Can you work these out from the drawing? Everything is in mm from the part's minimum corner. Give positions to 0.01 mm unless a question says otherwise; leave off trailing zeros. Write each loop counter-clockwise with the first axis right and the second up, starting at its lowest first coordinate (ties: lowest second). Pieces come first, ordered by that corner, then holes. Notation, with made-up numbers: (-3, 71) -> (27, 71) arc R21 ccw to (27, 92) -> close; hole circle Ø11 at (18.5, 59). An arc over 180 degrees is marked (long way). Use one line per item in the form item = value.
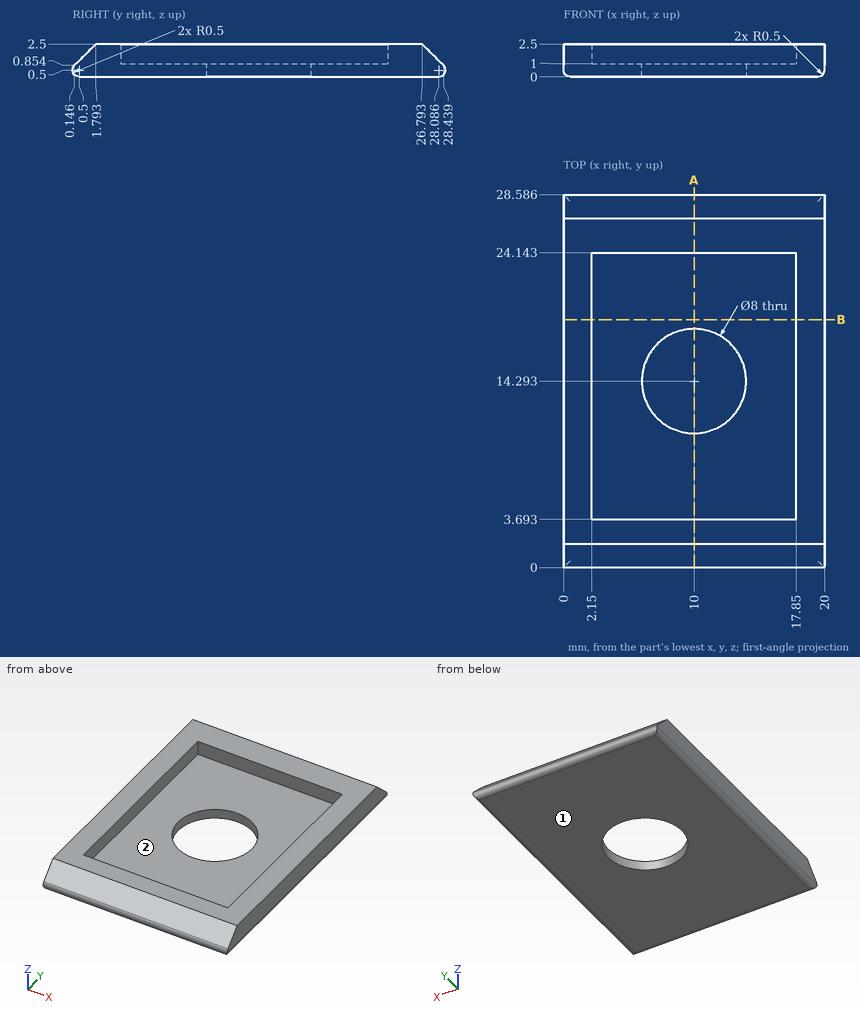
Q1. If we mould it in two halves opening along X, with no side actions, what happens to the marked faces 1 and 2? For each: +X half, -X half, draft (parallel to the pull), parting line (faces both ways), or undercut.
Result set:
face_1 = draft
face_2 = undercut
Q2. If I drill on line 1 along X through (y, z) = (7.75, 1.4); line 2 along Y through (x, z) = (10, 0.45); line 3 along Y through (x, z) = (10, 0.85) (1 decimal), over which ranges is the centre line in solid material (lowest first)? Write a range as from..to.
Result set:
line_1 = 0..2.15, 17.85..20
line_2 = 0..10.29, 18.29..28.58
line_3 = 0.1..10.3, 18.3..28.4
Q3. Will these pins go through, and if not, where does the flat tip stop? pin 1 Ø4.5 at (x, y) = (13.5, 12.5) entering from +Z; pin 2 Ø12 at (x, y) = (4.5, 14.5) entering from -Z.
Result set:
pin_1 = 1
pin_2 = 0
Q4. I want a section at B-B, the plane y = 19. Write out the boundary of the cut face in (x, z).
Result set:
outline = (0, 0.5) arc R0.5 ccw to (0.5, 0) -> (19.5, 0) arc R0.5 ccw to (20, 0.5) -> (20, 2.5) -> (17.85, 2.5) -> (17.85, 1) -> (2.15, 1) -> (2.15, 2.5) -> (0, 2.5) -> close
Q5. I want a section at A-A, the plane x = 10. Write out the boundary of the cut face in (y, z) (1 decimal).
Result set:
outline = (0.1, 0.9) arc R0.5 ccw to (0.5, 0) -> (10.3, 0) -> (10.3, 1) -> (3.7, 1) -> (3.7, 2.5) -> (1.8, 2.5) -> close; (18.3, 0) -> (28.1, 0) arc R0.5 ccw to (28.4, 0.9) -> (26.8, 2.5) -> (24.1, 2.5) -> (24.1, 1) -> (18.3, 1) -> close
